Check sheet for the modelled part. Datum: model origin and axes. Units: mm. A direction names the side the tool comes from. Round coordinates to 2 decimals unless told otherwise and drop trailing zeros. Loops run counter-clockwise (first coordinate to the right, second up) from the corner with the lowest first, then second, coordinate; pieces in that order, holes last. Notation, with made-up numbers: M -39.5,-3 L 14.5,-3 A10 ccw 14.5,12 Z; hole C 19.5,45 d11. An arc over 180 degrees is marked long. One line per question, with ' | ' between items. Start each with the question number.
(1) Section check C-C (y = 58). Record the boundary of the cut face in (x, z), and give its area (3 significant figures).
(2) Tool access check on faces 1 (the face through (-406.4, -2, 41)), 2 (the face through (425.45, -2, 41)). Record the directions out of +Z, -Z, +X, -X, +Y, -Y that give a thin tool (end or side, any length) a straight path to the whole face; none if there is none.
(3) Thickness scan on probe 1 along X at (y, z) = (-7, 12); probe 2 along Y at (x, z) = (-293, 74) (3 decimals). Record the ranges inside material, lowest first. Write a range as [from, to].
(4) Draft check along X on faces 3 (the face through (-425.45, -2, 41)), 4 (the face through (312, -117.475, 41)), 5 (the face through (-6, 136.525, 41)), 6 (the face through (-214.483, -2, 42)). Enter one of: +X half, -X half, draft (parallel to the pull), parting line (faces both ways), or undercut.
(5) Section check A-A (z = 24). Record the boundary of the cut face in (x, y) (3 decimals), and give its area (3 significant figures).
(6) Section check B-B (x = 145.5). Record the boundary of the cut face in (y, z) (3 decimals).
```python
from build123d import *

# Parameters (mm, degrees)
F1_W     = 850.9
F1_H     = 273.05
F1_W_2   = 812.8
F1_H_2   = 234.95
F2_DEPTH = 82.55
F3_W     = 19.05
F3_H     = 234.95
F4_DEPTH = 82.55
F5_W     = 19.05
F5_H     = 234.95
F6_DEPTH = 82.55
F7_W     = 19.05
F7_H     = 234.95
F8_DEPTH = 82.55


with BuildPart() as f2:
    # F1 (on face) → F2 (new body)
    with BuildSketch(Plane.XY):
        Rectangle(F1_W, F1_H)
        Rectangle(F1_W_2, F1_H_2, mode=Mode.SUBTRACT)
    extrude(amount=F2_DEPTH)

    # F3 (on face) → F4 (join)
    with BuildSketch(Plane.XY.offset(82.55)):
        with Locations((6.0091395862, 0)):
            Rectangle(F3_W, F3_H)
    extrude(amount=-F4_DEPTH)

    # F5 (on face) → F6 (join)
    with BuildSketch(Plane.XY.offset(82.55)):
        with Locations((-204.9579302069, 0)):
            Rectangle(F5_W, F5_H)
    extrude(amount=-F6_DEPTH)

    # F7 (on face) → F8 (join)
    with BuildSketch(Plane.XY.offset(82.55)):
        with Locations((210.9670697931, 0)):
            Rectangle(F7_W, F7_H)
    extrude(amount=-F8_DEPTH)


solid = f2.part
```
The answers:
1) outline: M -425.45,0 L -406.4,0 L -406.4,82.55 L -425.45,82.55 Z; M -214.48,0 L -195.43,0 L -195.43,82.55 L -214.48,82.55 Z; M -3.52,0 L 15.53,0 L 15.53,82.55 L -3.52,82.55 Z; M 201.44,0 L 220.49,0 L 220.49,82.55 L 201.44,82.55 Z; M 406.4,0 L 425.45,0 L 425.45,82.55 L 406.4,82.55 Z | area: 7,860 mm²
2) face 1: +Z, -Z | face 2: +Z, -Z, +X, +Y, -Y
3) probe 1: [-425.45, -406.4], [-214.48, -195.43], [-3.52, 15.53], [201.44, 220.49], [406.4, 425.45] | probe 2: [-136.525, -117.475], [117.475, 136.525]
4) face 3: -X half | face 4: undercut | face 5: draft | face 6: undercut
5) outline: M -425.45,-136.525 L 425.45,-136.525 L 425.45,136.525 L -425.45,136.525 Z; hole M -406.4,-117.475 L -214.483,-117.475 L -214.483,117.475 L -406.4,117.475 Z; hole M -195.433,-117.475 L -3.516,-117.475 L -3.516,117.475 L -195.433,117.475 Z; hole M 15.534,-117.475 L 201.442,-117.475 L 201.442,117.475 L 15.534,117.475 Z; hole M 220.492,-117.475 L 406.4,-117.475 L 406.4,117.475 L 220.492,117.475 Z | area: 54,800 mm²
6) outline: M -136.525,0 L -117.475,0 L -117.475,82.55 L -136.525,82.55 Z; M 117.475,0 L 136.525,0 L 136.525,82.55 L 117.475,82.55 Z
